Verification items for the finished model (mm, model axes). A direction names the side the tool comes from. Coordinates: 2 decimals unless noted, no trailing zeros. Order: outer loops, then holes, each group sorted by start corner. A loop starts at its lowest first (then second) coordinate and runs counter-clockwise, first axis right, second up. Notation, with made-up numbers: M -15.75,-18 L -5.75,-18 A17 ccw -5.75,-10 Z; hole C 85,30.25 d10. An arc over 180 degrees is marked long. Write item = value, one per line.
```python
from build123d import *

# Parameters (mm, degrees)
SKETCH1_W           = 75
SKETCH1_H           = 72.5
BOSS_EXTRUDE1_DEPTH = 10
CUT_EXTRUDE1_DEPTH  = 10
SKETCH3_W           = 75
SKETCH3_H           = 10
FEET_DEPTH          = 20
SKETCH4_R           = 3
FEET_HOLE_DEPTH     = 10
SKETCH6_W           = 8
SKETCH6_H           = 15
BOSS_EXTRUDE2_DEPTH = 18
CUT_EXTRUDE2_DEPTH  = 97.687641403
SKETCH5_R           = 4
SKETCH5_R_2         = 10
SKETCH5_R_3         = 9.124733902
CUT_EXTRUDE3_DEPTH  = 9.8
FILLET1_R           = 5
FILLET2_R           = 15


with BuildPart() as part:
    # Sketch1 → Boss-Extrude1 (new body)
    with BuildSketch(Plane.XY):
        with Locations((37.5, 36.25)):
            Rectangle(SKETCH1_W, SKETCH1_H)
    extrude(amount=BOSS_EXTRUDE1_DEPTH)

    # Sketch2 → Cut-Extrude1 (cut)
    with BuildSketch(Plane.XY.offset(10)):
        with BuildLine():
            Line((60, 65), (60, 72.5))
            Line((60, 72.5), (15, 72.5))
            Line((15, 72.5), (15, 65))
            ThreePointArc((15, 65), (37.5, 42.5), (60, 65))
        make_face()
    extrude(amount=-CUT_EXTRUDE1_DEPTH, mode=Mode.SUBTRACT)

    # Sketch3 → feet (add)
    with BuildSketch(Plane.XY.offset(10)):
        with Locations((37.5, 5)):
            Rectangle(SKETCH3_W, SKETCH3_H)
    extrude(amount=FEET_DEPTH)

    # Sketch4 → feet-hole (cut)
    with BuildSketch(Plane.XZ):
        with Locations(Location((7.5, 20, 0), (0, 0, 270))):
            Circle(SKETCH4_R)
        with Locations(Location((67.5, 20, 0), (0, 0, 270))):
            Circle(SKETCH4_R)
        with Locations(Location((37.5, 20, 0), (0, 0, 270))):
            Circle(SKETCH4_R)
    extrude(amount=-FEET_HOLE_DEPTH, mode=Mode.SUBTRACT)

    # Sketch6 → Boss-Extrude2 (add)
    with BuildSketch(Plane.XY.offset(10)):
        with Locations((22.5, 17.5)):
            Rectangle(SKETCH6_W, SKETCH6_H)
        with Locations((52.5, 17.5)):
            Rectangle(SKETCH6_W, SKETCH6_H)
    extrude(amount=BOSS_EXTRUDE2_DEPTH)

    # Sketch7 → Cut-Extrude2 (cut, through all)
    with BuildSketch(Plane.ZY.offset(-18.5)):
        Polygon((10, 25), (28, 10), (28, 25), align=None)
    extrude(amount=-CUT_EXTRUDE2_DEPTH, mode=Mode.SUBTRACT)

    # Sketch5 → Cut-Extrude3 (cut)
    with BuildSketch(Plane.XY.offset(10)):
        with Locations((7.5, 65)):
            Circle(SKETCH5_R)
        with Locations(Location((67.5, 65, 0), (0, 0, 180))):
            Circle(SKETCH5_R)
        with Locations((37.5, 25)):
            Circle(SKETCH5_R_2)
        with Locations((12.51923423, 36.579255476)):
            Circle(SKETCH5_R_3)
        with Locations(Location((62.48076577, 36.579255476, 0), (0, 0, 180))):
            Circle(SKETCH5_R_3)
    extrude(amount=-CUT_EXTRUDE3_DEPTH, mode=Mode.SUBTRACT)

    # Fillet1
    fillet1_edges = [part.edges().sort_by_distance(p)[0] for p in [
        (0, 72.5, 5),
        (15, 72.5, 5),
        (60, 72.5, 5),
        (75, 72.5, 5),
    ]]
    fillet(fillet1_edges, radius=FILLET1_R)

    # Fillet2
    fillet2_edges = [part.edges().sort_by_distance(p)[0] for p in [
        (0, 5, 30),
        (75, 5, 30),
    ]]
    fillet(fillet2_edges, radius=FILLET2_R)


solid = part.part
```
Item 1: Release check for a two-part mould opening along Y. For faces 1 (the flat face through (63, 36, 0.2)), 2 (the flat face through (22.444, 17.605, 18.874)), 3 (the flat face through (37, 29, 0)) record: pulls with the +Y half, pulls with the -Y half, needs draft (parallel to the pull), parting line crosses it, or undercut.
Report:
face_1 = undercut
face_2 = pulls with the +Y half
face_3 = needs draft
Item 2: Sectioned sample at C-C, the plane z = 7. Enter the section's corners in (x, y), then the cut area to 3 significant figures.
Report:
outline = M 0,0 L 75,0 L 75,67.5 A5 ccw 70,72.5 L 65,72.5 A5 ccw 60,67.5 L 60,65 A22.5 cw 15,65 L 15,67.5 A5 ccw 10,72.5 L 5,72.5 A5 ccw 0,67.5 Z; hole C 12.52,36.58 d18.25; hole C 7.5,65 d8; hole C 37.5,25 d20; hole C 62.48,36.58 d18.25; hole C 67.5,65 d8
area = 3,350 mm^2
Item 3: Sectioned sample at A-A, the plane x = 37.5. Enter the section's corners in (y, z), then the cut area to 3 significant figures.
Report:
outline = M 0,0 L 42.5,0 L 42.5,10 L 35,10 L 35,0.2 L 15,0.2 L 15,10 L 10,10 L 10,17 L 0,17 Z; M 0,23 L 10,23 L 10,30 L 0,30 Z
area = 369 mm^2
Item 4: Scan lines: L1, parallel to Y at x = 7, z = 3; L2, parallel to X at y = 42, z = 9.5; L3, parallel to Z at x = 65, y = 43.5. Record each from-to range of solid material in increasing order. Write a range as from..to.
Report:
L1 = 0..29.31, 43.85..61.03, 68.97..72.5
L2 = 0..5.18, 19.86..55.14, 69.82..75
L3 = 0..0.2
Item 5: Gauge pin test, flat ends, axial feed: pin 1 (10 mm diameter, centred on x = 48, y = 58, fed in from +Z); pin 2 (14.5 mm diameter, centred on x = 11.5, y = 34.5, fed in from +Z); pin 3 (12 mm diameter, centred on y = 15.5, z = 19.5, fed in from +X); pin 4 (12 mm diameter, centred on y = 14.5, z = 20.5, fed in from -X). Record the tip position at first contact, or that the pin passes through.
Report:
pin_1 = through
pin_2 = 10
pin_3 = 74.85
pin_4 = 0.08
Item 6: Sectioned sample at D-D, the plane x = 66.5. Enter the section's corners in (y, z).
Report:
outline = M 0,0 L 72.5,0 L 72.5,10 L 68.87,10 L 68.87,0.2 L 61.13,0.2 L 61.13,10 L 44.77,10 L 44.77,0.2 L 28.39,0.2 L 28.39,10 L 10,10 L 10,17.17 L 0,17.17 Z; M 0,22.83 L 10,22.83 L 10,28.52 L 0,28.52 Z
Item 7: Tool access check on faces 4 (the cylindrical face through (61.43, 71, 4.93)), 5 (the cylindrical face through (36.198, 34.915, 5.169)), 6 (the flat face through (67, 72.5, 5)). Record the directions out of +Z, -Z, +X, -X, +Y, -Y that give a thin tool (end or side, any length) a straight path to the whole face; none if there is none.
Report:
face_4 = +Z, -Z, +Y
face_5 = +Z
face_6 = +Z, -Z, +X, -X, +Y
Item 8: Sectioned sample at B-B, the plane z = 20. Enter the section's corners in (x, y), then the cut area to 3 significant figures.
Report:
outline = M 0.86,0 L 4.5,0 L 4.5,10 L 0.86,10 Z; M 10.5,0 L 34.5,0 L 34.5,10 L 26.5,10 L 26.5,16.67 L 18.5,16.67 L 18.5,10 L 10.5,10 Z; M 40.5,0 L 64.5,0 L 64.5,10 L 56.5,10 L 56.5,16.67 L 48.5,16.67 L 48.5,10 L 40.5,10 Z; M 70.5,0 L 74.14,0 L 74.14,10 L 70.5,10 Z
area = 660 mm^2
